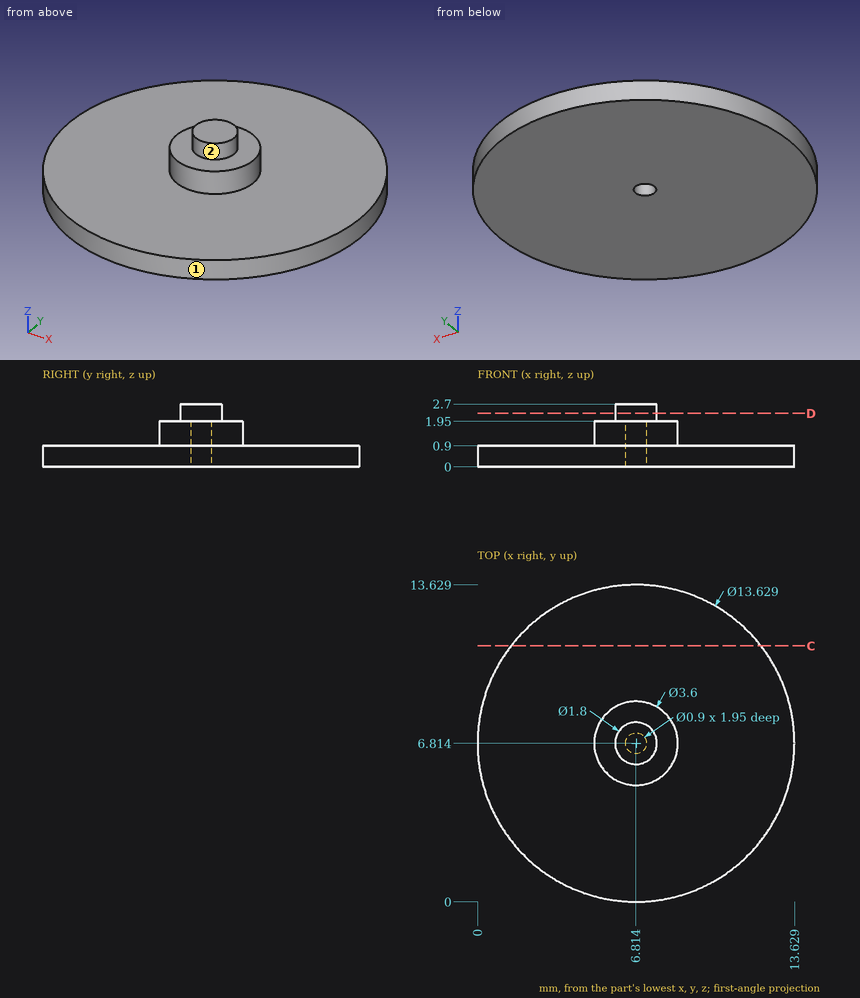
Could you check a few things on this drawing? It's one solid part, dimensions in mm from its lowest x, y, z. A direction names the side the tool comes from. Coordinates: 2 decimals unless noted, no trailing zeros. Order: outer loops, then holes, each group sorted by start corner. A loop starts at its lowest first (then second) coordinate and runs counter-clockwise, first axis right, second up. Notation, with made-up numbers: (69, -26.75) - (79, -26.75) arc R14 cw to (79, 0.25) - close; hole circle Ø5 at (54, -9.75). An arc over 180 degrees is marked (long way). Answer as a JSON object with one key per item and string values. Group by question number.
Q1. On a 3-axis mill with a long thin cutter (end or side, diameter ignored), from which of +Z, -Z, +X, -X, +Y, -Y can I reach the whole of each face in a straight line? I mean the marked faces 1 and 2. Say none if no direction works.
Q2. Imagine slicing it at D-D (z = 2.3). Please give me the cut outline in (x, y) (1 decimal).
Q3. I need wall thicknesses on line 1 (Z direction, x = 8.75, y = 13); line 2 (Y direction, x = 7.75, z = 0.8) (1 decimal); line 3 (X direction, y = 6.5, z = 1.1) (1 decimal). Which ranges of each line are inside material? Lowest first, please. Write a range as from..to.
Q4. Will these pins go through, and if not, where does the flat tip stop? P1, Ø1.5, axis at x = 11, z = 1.5, coming from the +Y side (1 decimal); P2, Ø1, axis at x = 4.5, z = 0.5, coming from the -Y side.
Q5. Imagine slicing it at C-C (y = 11). Please give me the cut outline in (x, z).
Determined:
{
 "1": {"face 1": "+Z, -Z", "face 2": "+Z"},
 "2": {"outline": "circle Ø1.8 at (6.8, 6.8)"},
 "3": {"line 1": "z = 0..0.9", "line 2": "y = 0.1..13.6", "line 3": "x = 5..6.5, 7.1..8.6"},
 "4": {"P1": "stops at y = 12.5", "P2": "stops at y = 0.25"},
 "5": {"outline": "(1.44, 0) - (12.19, 0) - (12.19, 0.9) - (1.44, 0.9) - close"}
}
